```python
from build123d import *

# Parameters (mm, degrees)
SKETCH3_R           = 1.5
BOSS_EXTRUDE3_DEPTH = 2
CUT_EXTRUDE1_DEPTH  = 3
FILLET1_R           = 2


with BuildPart() as part:
    # Sketch3 → Boss-Extrude3 (new body)
    with BuildSketch(Plane(origin=(0, 0, 0), x_dir=(1, 0, 0), z_dir=(0, 1, 0))):
        with BuildLine():
            Line((-9.26926183, -10.650603484), (-9.26926183, -17.650603484))
            Line((-9.26926183, -17.650603484), (9.73073817, -17.650603484))
            Line((9.73073817, -17.650603484), (9.73073817, -10.650603484))
            Line((9.73073817, -10.650603484), (31.167436549, -10.650603484))
            Line((31.167436549, -10.650603484), (31.167436549, -14.650603484))
            Line((31.167436549, -14.650603484), (37.167436549, -14.650603484))
            Line((37.167436549, -14.650603484), (37.167436549, -10.650603484))
            ThreePointArc((37.167436549, -10.650603484), (44.48073817, 5.599396516), (37.167436549, 21.849396516))
            Line((37.167436549, 21.849396516), (37.167436549, 25.849396516))
            Line((37.167436549, 25.849396516), (31.167436549, 25.849396516))
            Line((31.167436549, 25.849396516), (31.167436549, 21.849396516))
            Line((31.167436549, 21.849396516), (9.73073817, 21.849396516))
            Line((9.73073817, 21.849396516), (9.73073817, 31.849396516))
            Line((9.73073817, 31.849396516), (-9.26926183, 31.849396516))
            Line((-9.26926183, 31.849396516), (-9.26926183, 21.849396516))
            Line((-9.26926183, 21.849396516), (-30.705960209, 21.849396516))
            Line((-30.705960209, 21.849396516), (-30.705960209, 25.849396516))
            Line((-30.705960209, 25.849396516), (-36.705960209, 25.849396516))
            Line((-36.705960209, 25.849396516), (-36.705960209, 21.849396516))
            ThreePointArc((-36.705960209, 21.849396516), (-44.01926183, 5.599396516), (-36.705960209, -10.650603484))
            Line((-36.705960209, -10.650603484), (-36.705960209, -14.650603484))
            Line((-36.705960209, -14.650603484), (-30.705960209, -14.650603484))
            Line((-30.705960209, -14.650603484), (-30.705960209, -10.650603484))
            Line((-30.705960209, -10.650603484), (-9.26926183, -10.650603484))
        make_face()
        with Locations(Location((-33.705960209, 22.349396516, 0), (0, 0, 270))):
            Circle(SKETCH3_R, mode=Mode.SUBTRACT)
        with Locations(Location((-33.705960209, -11.150603484, 0), (0, 0, 270))):
            Circle(SKETCH3_R, mode=Mode.SUBTRACT)
        with Locations(Location((34.167436549, -11.150603484, 0), (0, 0, 270))):
            Circle(SKETCH3_R, mode=Mode.SUBTRACT)
        with Locations(Location((34.167436549, 22.349396516, 0), (0, 0, 270))):
            Circle(SKETCH3_R, mode=Mode.SUBTRACT)
        with Locations(Location((0.23073817, -14.150603484, 0), (0, 0, 270))):
            Circle(SKETCH3_R, mode=Mode.SUBTRACT)
        with Locations(Location((0.23073817, 28.349396516, 0), (0, 0, 270))):
            Circle(SKETCH3_R, mode=Mode.SUBTRACT)
    extrude(amount=BOSS_EXTRUDE3_DEPTH)

    # Sketch4 → Cut-Extrude1 (cut)
    with BuildSketch(Plane(origin=(0, 2, 0), x_dir=(1, 0, 0), z_dir=(0, 1, 0))):
        with BuildLine():
            Line((-25.01926183, 10.599396516), (-9.01926183, 10.599396516))
            ThreePointArc((-9.01926183, 10.599396516), (-4.01926183, 5.599396516), (-9.01926183, 0.599396516))
            Line((-9.01926183, 0.599396516), (-25.01926183, 0.599396516))
            ThreePointArc((-25.01926183, 0.599396516), (-30.01926183, 5.599396516), (-25.01926183, 10.599396516))
        make_face()
    extrude(amount=-CUT_EXTRUDE1_DEPTH, mode=Mode.SUBTRACT)

    # Fillet1
    fillet1_edges = [part.edges().sort_by_distance(p)[0] for p in [
        (-30.705960209, 1, 14.650603484),
        (-36.705960209, 1, 14.650603484),
        (-36.705960209, 1, -25.849396516),
        (-30.705960209, 1, -25.849396516),
        (-9.26926183, 1, -31.849396516),
        (9.73073817, 1, -31.849396516),
        (31.167436549, 1, -25.849396516),
        (37.167436549, 1, -25.849396516),
        (37.167436549, 1, 14.650603484),
        (31.167436549, 1, 14.650603484),
        (9.73073817, 1, 17.650603484),
        (-9.26926183, 1, 17.650603484),
    ]]
    fillet(fillet1_edges, radius=FILLET1_R)


solid = part.part
```
Could you check a few things on this model? Use its own coordinates, in mm. A direction names the side the tool comes from. Round coordinates to 2 decimals unless told otherwise and drop trailing zeros. Write each loop counter-clockwise with the first axis right and the second up, starting at its lowest first coordinate (ties: lowest second). Pieces come first, ordered by that corner, then holes.
(1) For pin 1 (1.8 mm diameter, centred on x = 0.23, z = -28.35, fed in from +Y); pin 2 (0.6 mm diameter, centred on x = 34, y = 1, fed in from -Z); pin 3 (0.6 mm diameter, centred on x = -18.5, y = 1, fed in from +Z); pin 4 (0.6 mm diameter, centred on y = 1, z = -22.5, fed in from +X), each with a flat end and sliding along its axis, tell me the tip position at first contact or that it passes through.
Findings below:
pin 1: passes through
pin 2: stops at z = -25.85
pin 3: stops at z = 10.65
pin 4: stops at x = 37.17
(2) If I drill on probe 1 along Z at (x, y) = (-20.5, 1.55); probe 2 along X at (y, z) = (0.85, -22); probe 3 along Z at (x, y) = (33.5, 1.25), over which ranges is the centre line in solid material (lowest first)?
Findings below:
probe 1: z = -21.85 to -10.6, -0.6 to 10.65
probe 2: x = -36.71 to -35.16, -32.25 to -30.71, -9.27 to 9.73, 31.17 to 32.71, 35.63 to 37.17
probe 3: z = -25.85 to -23.69, -21.01 to 9.81, 12.49 to 14.65
(3) Suppose I cut it at B-B on z = -13.5. Write out the boundary of the cut face in (x, y), and give its area (3 significant figures).
Findings below:
outline: (-42.53, 0) - (42.99, 0) - (42.99, 2) - (-42.53, 2) - close
area: 171 mm2
(4) Thinking about a two-plate mould opening in X: for faces 1 (the face through (-34, 1, 14.651)), 2 (the face through (20, 1, 10.651)), 3 (the face through (37.167, 1, -23)), which applies, +X half, -X half, draft (parallel to the pull), parting line (faces both ways), or undercut?
Findings below:
face 1: draft
face 2: undercut
face 3: +X half
(5) Suppose I cut it at A-A on x = 24.5. Write out the boundary of the cut face in (y, z), and give its area (3 significant figures).
Findings below:
outline: (0, -21.85) - (2, -21.85) - (2, 10.65) - (0, 10.65) - close
area: 65.0 mm2
(6) Suppose I cut it at C-C on y = 0.5. State how many separate pieces and enclosed holes the cut face has, and give its area (3 significant figures).
Findings below:
separate pieces: 1
enclosed holes: 7
area: 2,860 mm2
(7) Which directions (+Z, -Z, +X, -X, +Y, -Y) give clear straight access to the entire face, cutting with the end or side of a thin tool? Please do faces 4 (the face through (-17, 1, -10.599)), 5 (the face through (-36.706, 1, 12)), 6 (the face through (21, 1, -21.849)), 7 (the face through (34, 1, 14.651)), 8 (the face through (31.167, 1, 12)).
Findings below:
face 4: +Y, -Y
face 5: +Z, -X, +Y, -Y
face 6: -Z, +Y, -Y
face 7: +Z, +X, +Y, -Y
face 8: +Z, +Y, -Y
